from build123d import *

# Parameters (mm, degrees)
F0_W     = 35
F0_H     = 35
F0_R     = 1.5
F1_DEPTH = 3
F3_DEPTH = 3
F5_DEPTH = 25


with BuildPart() as f1:
    # F0 (on Top) → F1 (new body)
    with BuildSketch(Plane.XY):
        Rectangle(F0_W, F0_H)
        with Locations((-13, -13)):
            Circle(F0_R, mode=Mode.SUBTRACT)
        with Locations((13, -13)):
            Circle(F0_R, mode=Mode.SUBTRACT)
        with Locations((-13, 13)):
            Circle(F0_R, mode=Mode.SUBTRACT)
        with BuildLine():
            ThreePointArc((0, 12), (8.485281, 8.485281), (12, 0))
            ThreePointArc((12, 0), (-8.485281, -8.485281), (0, 12))
        make_face(mode=Mode.SUBTRACT)
        with Locations((13, 13)):
            Circle(F0_R, mode=Mode.SUBTRACT)
    extrude(amount=F1_DEPTH)

    # F2 (on face) → F3 (join)
    with BuildSketch(Plane.XY.offset(3)):
        Polygon((17.5, 17.5), (17.5, 32.5), (-32.5, 32.5), (-32.5, -17.5), (-17.5, -17.5), (-17.5, 17.5), align=None)
    extrude(amount=-F3_DEPTH)

    # F4 (on face) → F5 (cut)
    with BuildSketch(Plane.XY.offset(3)):
        with BuildLine():
            ThreePointArc((13, 23.5), (14.06066, 23.93934), (14.5, 25))
            Line((14.5, 25), (13, 25))
            Line((13, 25), (13, 23.5))
        make_face()
        with BuildLine():
            Line((13, 25), (14.5, 25))
            ThreePointArc((14.5, 25), (13, 26.5), (11.5, 25))
            Line((11.5, 25), (13, 25))
        make_face()
        with BuildLine():
            ThreePointArc((-23.5, -13), (-23.93934, -11.93934), (-25, -11.5))
            Line((-25, -11.5), (-25, -13))
            Line((-25, -13), (-23.5, -13))
        make_face()
        with BuildLine():
            Line((-25, -13), (-25, -11.5))
            ThreePointArc((-25, -11.5), (-26.5, -13), (-25, -14.5))
            Line((-25, -14.5), (-25, -13))
        make_face()
        with BuildLine():
            ThreePointArc((-23.5, 6), (-23.93934, 7.06066), (-25, 7.5))
            Line((-25, 7.5), (-25, 4.5))
            ThreePointArc((-25, 4.5), (-23.93934, 4.93934), (-23.5, 6))
        make_face()
        with BuildLine():
            Line((-25, 4.5), (-25, 7.5))
            ThreePointArc((-25, 7.5), (-26.5, 6), (-25, 4.5))
        make_face()
        with BuildLine():
            ThreePointArc((-25, 23.5), (-23.93934, 23.93934), (-23.5, 25))
            Line((-23.5, 25), (-25, 25))
            Line((-25, 25), (-25, 23.5))
        make_face()
        with BuildLine():
            Line((-25, 25), (-23.5, 25))
            ThreePointArc((-23.5, 25), (-26.06066, 26.06066), (-25, 23.5))
            Line((-25, 23.5), (-25, 25))
        make_face()
        with BuildLine():
            ThreePointArc((-7.5, 25), (-6, 23.5), (-4.5, 25))
            Line((-4.5, 25), (-7.5, 25))
        make_face()
        with BuildLine():
            Line((-7.5, 25), (-4.5, 25))
            ThreePointArc((-4.5, 25), (-6, 26.5), (-7.5, 25))
        make_face()
        with BuildLine():
            Line((13, 23.5), (13, 25))
            Line((13, 25), (11.5, 25))
            ThreePointArc((11.5, 25), (11.93934, 23.93934), (13, 23.5))
        make_face()
        with BuildLine():
            Line((-23.5, -13), (-25, -13))
            Line((-25, -13), (-25, -14.5))
            ThreePointArc((-25, -14.5), (-23.93934, -14.06066), (-23.5, -13))
        make_face()
    extrude(amount=-F5_DEPTH, mode=Mode.SUBTRACT)


solid = f1.part
Check sheet for the modelled part. Datum: model origin and axes. Units: mm. Round coordinates to 2 decimals unless told otherwise and drop trailing zeros. Loops run counter-clockwise (first coordinate to the right, second up) from the corner with the lowest first, then second, coordinate; pieces in that order, holes last. Notation, with made-up numbers: M 80.25,25.5 L 126.25,25.5 A27 cw 126.25,45.5 Z; hole C 19,82.25 d8. An arc over 180 degrees is marked long. One line per item, written item: value.
(1) Depth check by flat-ended pin: pin 1 Ø3.5 at (x, y) = (-6, 25) entering from +Z; pin 2 Ø5 at (x, y) = (-7, -4.5) entering from +Z. Enter the tip coordinate at first touch or a pass-through.
Computed values:
pin 1: stops at z = 3
pin 2: passes through
(2) Release check for a two-part mould opening along Y. For faces 1 (the face through (-8, 13, 3)), 2 (the face through (-7, 32.5, 2)), 3 (the face through (11.5, -12.93, 1.48)) record: +Y half, -Y half, draft (parallel to the pull), parting line (faces both ways), or undercut.
Computed values:
face 1: draft
face 2: +Y half
face 3: undercut
(3) Sectioned sample at D-D, the plane y = -7. Record the cut outline in (x, z), then the cut area to 3 significant figures.
Computed values:
outline: M -32.5,0 L -9.75,0 L -9.75,3 L -32.5,3 Z; M 9.75,0 L 17.5,0 L 17.5,3 L 9.75,3 Z
area: 91.5 mm^2
(4) Sectioned sample at B-B, the plane x = 10.5. Record the cut outline in (y, z).
Computed values:
outline: M -17.5,0 L -5.81,0 L -5.81,3 L -17.5,3 Z; M 5.81,0 L 32.5,0 L 32.5,3 L 5.81,3 Z
(5) Thickness scan on line 1 (Y direction, x = -25, z = 0.9); line 2 (Y direction, x = -13, z = 1.65); line 3 (X direction, y = 0, z = 0.8). Record the ranges inside material, lowest first.
Computed values:
line 1: y = -17.5 to -14.5, -11.5 to 4.5, 7.5 to 23.5, 26.5 to 32.5
line 2: y = -17.5 to -14.5, -11.5 to 11.5, 14.5 to 32.5
line 3: x = -32.5 to -12, 12 to 17.5
(6) Sectioned sample at C-C, the plane z = 0.55. Count the separate pieces of the cut face and the enclosed holes in it, then the cut area to 3 significant figures.
Computed values:
separate pieces: 1
enclosed holes: 10
area: 1,980 mm^2
(7) Sectioned sample at A-A, the plane x = -13. Record the cut outline in (y, z).
Computed values:
outline: M -17.5,0 L -14.5,0 L -14.5,3 L -17.5,3 Z; M -11.5,0 L 11.5,0 L 11.5,3 L -11.5,3 Z; M 14.5,0 L 32.5,0 L 32.5,3 L 14.5,3 Z
